```python
from build123d import *

# Parameters (mm, degrees)
F0_W      = 62.632754
F0_H      = 44.497188
F1_DEPTH  = 25.4
F2_R      = 9.609065
F3_DEPTH  = 142.494
F4_R      = 14.478505
F4_R_2    = 11.60909
F5_DEPTH  = 111.506
F6_R      = 9.726664
F7_DEPTH  = 125.476
F8_W      = 25.4
F8_H      = 29.555707
F9_DEPTH  = 112.776
F10_R     = 6.575743
F11_DEPTH = 201.168


with BuildPart() as f1:
    # F0 (on Right) → F1 (new body)
    with BuildSketch(Plane.YZ):
        with Locations((31.316377, -22.248594)):
            Rectangle(F0_W, F0_H)
    extrude(amount=F1_DEPTH)

    # F2 (on face) → F3 (join)
    with BuildSketch(Plane.XZ):
        with Locations((16.751623, -28.44735)):
            Circle(F2_R)
    extrude(amount=F3_DEPTH)

    # F4 (on face) → F5 (join)
    with BuildSketch(Plane.YZ.offset(25.4)):
        with Locations((27.960511, -23.682347)):
            Circle(F4_R)
        with Locations((27.960511, -23.682347)):
            Circle(F4_R_2, mode=Mode.SUBTRACT)
    extrude(amount=F5_DEPTH)

    # F6 (on face) → F7 (join)
    with BuildSketch(Plane(origin=(0, 0, 0), x_dir=(0, -1, 0), z_dir=(-1, 0, 0))):
        with Locations((-34.521122, -21.086203)):
            Circle(F6_R)
    extrude(amount=F7_DEPTH)

    # F8 (on face) → F9 (join)
    with BuildSketch(Plane(origin=(0, 62.632754, 0), x_dir=(-1, 0, 0), z_dir=(0, 1, 0))):
        with Locations((-12.7, -26.358702)):
            Rectangle(F8_W, F8_H)
    extrude(amount=F9_DEPTH)

    # F10 (on face) → F11 (join)
    with BuildSketch(Plane(origin=(0, 175.408754, 0), x_dir=(-1, 0, 0), z_dir=(0, 1, 0))):
        with Locations((-13.258439, -26.675297)):
            Circle(F10_R)
    extrude(amount=F11_DEPTH)


solid = f1.part
```
Could you check a few things on this model? Use its own coordinates, in mm. A direction names the side the tool comes from. Coordinates: 2 decimals unless noted, no trailing zeros. Write each loop counter-clockwise with the first axis right and the second up, starting at its lowest first coordinate (ties: lowest second). Pieces come first, ordered by that corner, then holes. Notation, with made-up numbers: (68.5, -9) -> (107.5, -9) arc R22 ccw to (107.5, 10) -> close; hole circle Ø1 at (70, -29.5). An arc over 180 degrees is marked (long way). Return JSON: item names as keys, results as strings.
(1) We'd pull the mould along Y, two halves only. Please class faces 1 (the cylindrical face through (80.37, 33.32, -33.98)), 2 (the flat face through (13, 62.633, -6)), 3 (the cylindrical face through (80.4, 13.5, -23)), 4 (the flat face through (25.4, 28, -24)): +Y half, -Y half, draft (parallel to the pull), parting line (faces both ways), or undercut.
Numbers:
{"face 1": "undercut", "face 2": "+Y half", "face 3": "parting line", "face 4": "undercut"}
(2) I'm going to push flat-ended pins straight in: pin 1 (8 mm diameter, centred on x = 35.5, z = -14, fed in from +Y); pin 2 (6 mm diameter, centred on x = 26, z = -14, fed in from +Y); pin 3 (2 mm diameter, centred on x = -48.5, z = -20.5, fed in from -Y). Where does each tip first touch, or does it pass through?
Numbers:
{"pin 1": "stops at y = 41.28", "pin 2": "stops at y = 175.41", "pin 3": "stops at y = 24.79"}
(3) Imagine slicing it at D-D, the plane x = -36. Please give me the cut outline in (y, z).
Numbers:
{"outline": "circle Ø19.45 at (34.52, -21.09)"}
(4) Which directions (+Z, -Z, +X, -X, +Y, -Y) give clear straight access to the entire face, cutting with the end or side of a thin tool? Please do faces 5 (the cylindrical face through (-61.86, 25.244, -18.165)), 6 (the cylindrical face through (14.67, -70.25, -37.83)), 7 (the flat face through (13, 118, -41.137)), 8 (the flat face through (7, 175.409, -23)).
Numbers:
{"face 5": "-X", "face 6": "-Y", "face 7": "-Z, +X, -X, +Y", "face 8": "+Y"}
(5) Imagine slicing it at A-A, the plane y = 169.5. Please give me the cut outline in (x, z), then the cut area to 3 significant figures.
Numbers:
{"outline": "(0, -41.14) -> (25.4, -41.14) -> (25.4, -11.58) -> (0, -11.58) -> close", "area": "751 mm2"}
(6) I need wall thicknesses on L1, parallel to X at y = 250.5, z = -26.5; L2, parallel to X at y = 61, z = -39; L3, parallel to Y at x = 19.5, z = -22. Which ranges of each line are inside material? Lowest first, please.
Numbers:
{"L1": "x = 6.69 to 19.83", "L2": "x = 0 to 25.4", "L3": "y = -142.49 to 175.41"}
(7) Imagine slicing it at B-B, the plane x = 69. Please give me the cut outline in (y, z).
Numbers:
{"outline": "circle Ø28.96 at (27.96, -23.68); hole circle Ø23.22 at (27.96, -23.68)"}
(8) Imagine slicing it at C-C, the plane y = 292. Please give me the cut outline in (x, z).
Numbers:
{"outline": "circle Ø13.15 at (13.26, -26.68)"}
